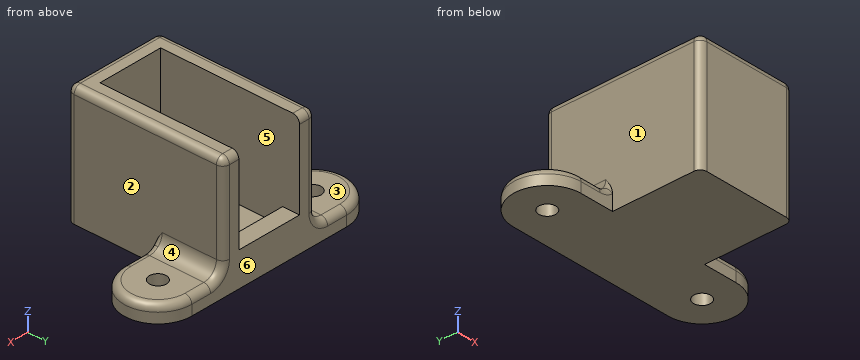
Autodesk Fusion 360 part; units mm, degrees
sketch "Sketch1" plane through (0, 0, 0) normal (0, 0, 1) x (1, 0, 0)
  line L0 (0, 0) -> (12.2682, 0)
  line L1 (12.2682, 0) -> (12.2682, 22.86)
  line L2 (12.2682, 22.86) -> (0, 22.86)
  line L3 (0, 22.86) -> (0, 0)
  line L4 (-3.175, -3.175) -> (15.4432, -3.175)
  line L5 (15.4432, -3.175) -> (15.4432, 26.035)
  line L6 (15.4432, 26.035) -> (-3.175, 26.035)
  line L7 (-3.175, 26.035) -> (-3.175, -3.175)
  line L8 (0, 22.86) -> (0, 26.035)
  line L9 (12.2682, 22.86) -> (12.2682, 26.035)
  dimension "d1" = 12.2682
  dimension "d2" = 22.86
  dimension "d3" = 3.175
extrude "Extrude1" add sketch "Sketch1" along normal blind 3.175
sketch "Sketch2" plane through (0, 0, 3.175) normal (0, 0, 1) x (-1, 0, 0)
  line L0 (3.175, -26.035) -> (3.175, 3.175)
  line L1 (3.175, 3.175) -> (-15.4432, 3.175)
  line L2 (-15.4432, 3.175) -> (-15.4432, -26.035)
  line L3 (-15.4432, -26.035) -> (3.175, -26.035)
  line L4 (-12.2682, 0) -> (-12.2682, -22.86)
  line L5 (-12.2682, -22.86) -> (0, -22.86)
  line L6 (0, -22.86) -> (0, 0)
  line L7 (0, 0) -> (-12.2682, 0)
  dimension "d6" = -3.175
extrude "Extrude2" add sketch "Sketch2" along normal blind 3.175
sketch "Sketch3" plane through (0, 0, 6.35) normal (0, 0, 1) x (-1, 0, 0)
  line L0 (-12.2682, 0) -> (0, 0)
  line L1 (0, 0) -> (0, -22.86)
  line L2 (0, -22.86) -> (-12.2682, -22.86)
  line L3 (-12.2682, -22.86) -> (-12.2682, 0)
  line L4 (-15.4432, -26.035) -> (3.175, -26.035)
  line L5 (3.175, -26.035) -> (3.175, 3.175)
  line L6 (3.175, 3.175) -> (-15.4432, 3.175)
  line L7 (-15.4432, 3.175) -> (-15.4432, -26.035)
  line L8 (0, -22.86) -> (0, -26.035)
  line L9 (-12.2682, -22.86) -> (-12.2682, -26.035)
extrude "Extrude3" add sketch "Sketch3" along normal blind 16.002 contours L0 L1 L3 L4 L5 L6 L7 L8 L9
sketch "Sketch4" plane through (0, 0, 0) normal (0, 0, -1) x (1, 0, 0)
  line L0 (-3.175, 3.175) -> (-3.175, -26.035)
  line L1 (-3.175, -26.035) -> (15.4432, -26.035)
  line L2 (15.4432, -26.035) -> (15.4432, 3.175)
  line L3 (15.4432, 3.175) -> (-3.175, 3.175)
  line L4 (15.4432, -26.035) -> (21.7932, -26.035)
  line L5 (21.7932, -26.035) -> (21.7932, -19.685)
  line L6 (21.7932, -19.685) -> (15.4432, -19.685)
  line L7 (15.4432, -19.685) -> (15.4432, -26.035)
  line L8 (-3.175, -26.035) -> (-9.525, -26.035)
  line L9 (-9.525, -26.035) -> (-9.525, -19.685)
  line L10 (-9.525, -19.685) -> (-3.175, -19.685)
  line L11 (-3.175, -19.685) -> (-3.175, -26.035)
  circle A0 centre (21.7932, -19.685) radius 6.35
  circle A1 centre (-9.525, -19.685) radius 6.35
  line L12 (-9.525, -19.685) -> (21.7932, -19.685)
  line L13 (21.7932, -19.685) -> (21.7932, -13.335)
  line L14 (21.7932, -13.335) -> (-9.525, -13.335)
  line L15 (-9.525, -13.335) -> (-9.525, -19.685)
  dimension "d11" = 6.35
  dimension "d12" = 6.35
  dimension "d13" = 6.35
  dimension "d14" = 6.35
extrude "Extrude4" add sketch "Sketch4" against normal blind 3.175 contours L0 A1 L14 | L9 L10 A1 L12 | L10 A1 L12 L15 | L0 L8 L11 A1 | L9 A1 L15 | L2 L4 L7 A0 | L6 A0 L12 L13 | L2 A0 L14 | L5 L6 A0 L12 | L5 A0 L13
sketch "Sketch5" plane through (0, 0, 3.175) normal (0, 0, 1) x (-1, 0, 0)
  line L0 (-15.4432, -26.035) -> (-15.4432, -13.335)
  line L1 (-15.4432, -13.335) -> (-21.7932, -13.335)
  arc A0 (-21.7932, -13.335) -> (-21.7932, -26.035) centre (-21.7932, -19.685) ccw
  line L2 (-21.7932, -26.035) -> (-15.4432, -26.035)
  circle A1 centre (-21.7932, -19.685) radius 1.5875
  dimension "d17" = 3.175
extrude "Extrude5" cut sketch "Sketch5" against normal blind 127 contours A1
sketch "Sketch6" plane through (0, 0, 3.175) normal (0, 0, 1) x (-1, 0, 0)
  arc A0 (9.525, -26.035) -> (9.525, -13.335) centre (9.525, -19.685) ccw
  line L0 (9.525, -13.335) -> (3.175, -13.335)
  line L1 (3.175, -13.335) -> (3.175, -26.035)
  line L2 (3.175, -26.035) -> (9.525, -26.035)
  circle A1 centre (9.525, -19.685) radius 1.5875
  dimension "d20" = 3.175
extrude "Extrude6" cut sketch "Sketch6" against normal blind 25.4 contours A1
fillet "Fillet1" radius 2.54 1 edges at (15.4432, 19.685, 3.175)
fillet "Fillet2" radius 2.54 1 edges at (-3.175, 19.685, 3.175)
fillet "Fillet3" radius 1.27 17 edges at (-3.175, 11.43, 22.352) (-3.9189, 13.335, 3.9189) (-7.62, 13.335, 3.175) (-15.875, 19.685, 3.175) (-7.62, 26.035, 3.175) (-3.9189, 26.035, 3.9189) (-3.175, 26.035, 14.0335) (-3.175, -3.175, 11.176) (15.4432, -3.175, 11.176) (6.1341, -3.175, 22.352) (15.4432, 11.43, 22.352) (16.1871, 13.335, 3.9189) (19.8882, 13.335, 3.175) (28.1432, 19.685, 3.175) (19.8882, 26.035, 3.175) (16.1871, 26.035, 3.9189) (15.4432, 26.035, 14.0335)
For this review, take the finished solid that the model builds, in its own axes (mm). Face numbers are marked on the shaded views. A direction names the side the tool comes from. Round coordinates to 2 decimals unless told otherwise and drop trailing zeros. Write each loop counter-clockwise with the first axis right and the second up, starting at its lowest first coordinate (ties: lowest second). Pieces come first, ordered by that corner, then holes. Notation, with made-up numbers: (55, -11.75) - (64, -11.75) arc R36 cw to (64, 24.25) - close; hole circle Ø8 at (-24.5, 10.5). An arc over 180 degrees is marked (long way). Use a Markdown table: item, result.
Q1. We need section B-B (x = -9). Give the boundary of the cut face in (y, z) (3 decimals).
Derived:
| item | result |
|---|---|
| outline | (13.335, 0) - (18.187, 0) - (18.187, 3.175) - (14.605, 3.175) arc R1.27 ccw to (13.335, 1.905) - close; (21.183, 0) - (26.035, 0) - (26.035, 1.905) arc R1.27 ccw to (24.765, 3.175) - (21.183, 3.175) - close |
Q2. We need section D-D (x = 9). Give the boundary of the cut face in (y, z) (3 decimals), plus the area to 3 significant figures.
Derived:
| item | result |
|---|---|
| outline | (-3.175, 0) - (26.035, 0) - (26.035, 6.35) - (22.86, 6.35) - (22.86, 3.175) - (0, 3.175) - (0, 22.352) - (-1.905, 22.352) arc R1.27 ccw to (-3.175, 21.082) - close |
| area | 163 mm2 |
Q3. We need section C-C (z = 11.5). Give the boundary of the cut face in (x, y) (3 decimals), plus the area to 3 significant figures.
Derived:
| item | result |
|---|---|
| outline | (-3.175, -1.905) arc R1.27 ccw to (-1.905, -3.175) - (14.173, -3.175) arc R1.27 ccw to (15.443, -1.905) - (15.443, 24.765) arc R1.27 ccw to (14.173, 26.035) - (12.268, 26.035) - (12.268, 0) - (0, 0) - (0, 26.035) - (-1.905, 26.035) arc R1.27 ccw to (-3.175, 24.765) - close |
| area | 223 mm2 |
Q4. Wall thickness on line 1 along X through (y, z) = (22.75, 6.5) (3 decimals); line 2 along Y through (x, z) = (2, 3.5) (3 decimals); line 3 along Z through (x, y) = (8, 22.75) (3 decimals): over which ranges is each line inside the solid? List them lowest first.
Derived:
| item | result |
|---|---|
| line 1 | x = -3.175 to 0, 12.268 to 15.443 |
| line 2 | y = -3.175 to 0, 22.86 to 26.035 |
| line 3 | z = 0 to 3.175 |
Q5. Clearance check with flat-ended pins moving along their axes: pin 1 (1.4 mm diameter, centred on x = -6.5, z = 1, fed in from -Y) (3 decimals); pin 2 (4.5 mm diameter, centred on x = 22.5, y = 21.5, fed in from +Z) (3 decimals); pin 3 (1.5 mm diameter, centred on x = -3.5, y = 16, fed in from +Z). State where each tip first meets the part, or that it passes through.
Derived:
| item | result |
|---|---|
| pin 1 | stops at y = 13.335 |
| pin 2 | stops at z = 3.175 |
| pin 3 | stops at z = 22.03 |
Q6. We need section A-A (y = 6). Give the boundary of the cut face in (x, z) (3 decimals).
Derived:
| item | result |
|---|---|
| outline | (-3.175, 0) - (15.443, 0) - (15.443, 21.082) arc R1.27 ccw to (14.173, 22.352) - (12.268, 22.352) - (12.268, 3.175) - (0, 3.175) - (0, 22.352) - (-1.905, 22.352) arc R1.27 ccw to (-3.175, 21.082) - close |
Q7. The part is to be moulded in two halves that separate along X. For the marked faces 4, 5 and 6, say which applies: pulls with the +X half, pulls with the -X half, needs draft (parallel to the pull), parting line crosses it, or undercut.
Derived:
| item | result |
|---|---|
| face 4 | pulls with the +X half |
| face 5 | undercut |
| face 6 | needs draft |
Q8. Machinability: for the marked faces 1, 2 and 3, which of the approach directions +Z, -Z, +X, -X, +Y, -Y give a long, thin tool a straight path to every point of the face, cutting with its end or side? Answer none if there is none.
Derived:
| item | result |
|---|---|
| face 1 | +Z, -X, -Y |
| face 2 | +Z, +X, -Y |
| face 3 | +Z, -X, +Y, -Y |
